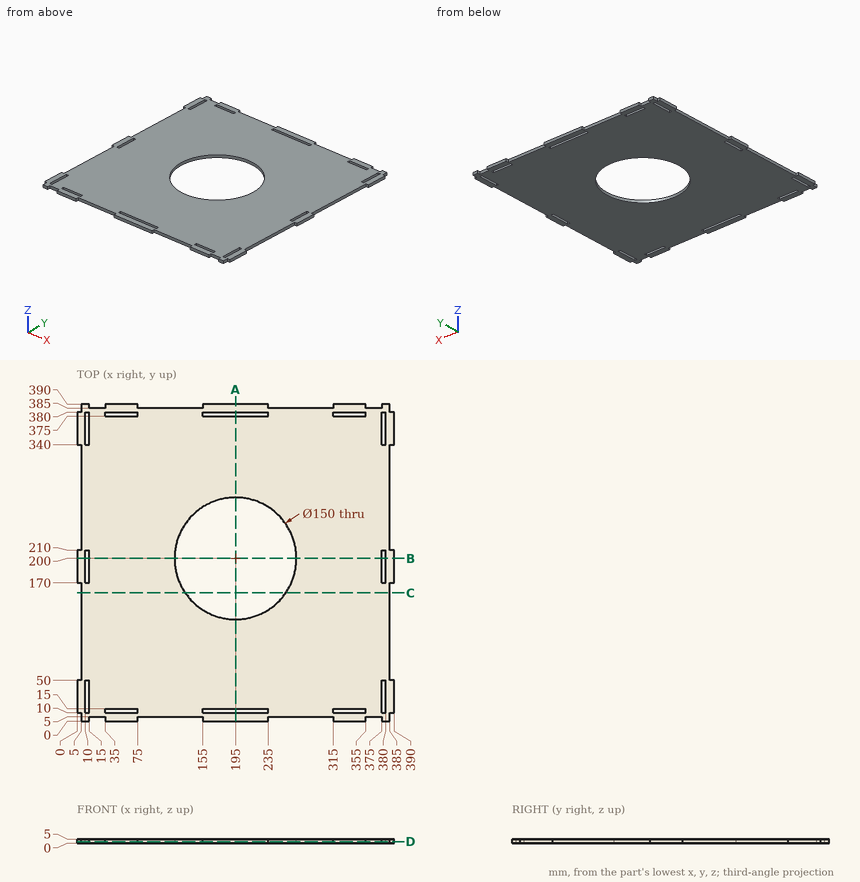
Source: three-view drawing plus pictorial views. Frame: mm from the lowest corner of the part. Round coordinates to 2 decimals unless told otherwise and drop trailing zeros. Loops run counter-clockwise (first coordinate to the right, second up) from the corner with the lowest first, then second, coordinate; pieces in that order, holes last.
Q1. Ray query, line 1 (Y direction, x = 195, z = 3.95); line 2 (Y direction, x = 328, z = 2.15); line 3 (Y direction, x = 216, z = 4.15). Return the intervals inside material, ascending.
Q2. Section D-D, the plane z = 1.9. State how many separate pieces and enclosed holes the cut face has, plus the area to 3 significant figures.
Q3. Section A-A, the plane x = 195. Return loops of the section in (y, z), plus the area to 3 significant figures.
Q4. First-contact query: P1, Ø1, axis at y = 246, z = 1.5, coming from the -X side; P2, Ø2.5, axis at x = 388.5, z = 2.5, coming from the +Y side; P3, Ø1, axis at x = 248, z = 1, coming from the +Y side. Flat tips, straight axial feed; report the tip coordinate or a pass-through.
Q5. Section B-B, the plane y = 200. Return loops of the section in (x, z), plus the area to 3 significant figures.
Q6. Section C-C, the plane y = 157.5. Return loops of the section in (x, z), plus the area to 3 significant figures.
Solutions:
1. line 1: y = 0 to 10, 15 to 125, 275 to 375, 380 to 390
1. line 2: y = 0 to 10, 15 to 375, 380 to 390
1. line 3: y = 0 to 10, 15 to 128, 272 to 375, 380 to 390
2. separate pieces: 1
2. enclosed holes: 13
2. area: 127,000 mm2
3. outline: (0, 0) - (10, 0) - (10, 5) - (0, 5) - close; (15, 0) - (125, 0) - (125, 5) - (15, 5) - close; (275, 0) - (375, 0) - (375, 5) - (275, 5) - close; (380, 0) - (390, 0) - (390, 5) - (380, 5) - close
3. area: 1,150 mm2
4. P1: stops at x = 5
4. P2: stops at y = 380
4. P3: stops at y = 385
5. outline: (0, 0) - (10, 0) - (10, 5) - (0, 5) - close; (15, 0) - (120, 0) - (120, 5) - (15, 5) - close; (270, 0) - (375, 0) - (375, 5) - (270, 5) - close; (380, 0) - (390, 0) - (390, 5) - (380, 5) - close
5. area: 1,150 mm2
6. outline: (5, 0) - (133.2, 0) - (133.2, 5) - (5, 5) - close; (256.8, 0) - (385, 0) - (385, 5) - (256.8, 5) - close
6. area: 1,280 mm2
